Check sheet for the drawn part. Datum: minimum x, y, z corner. Units: mm. A direction names the side the tool comes from. Round coordinates to 2 decimals unless told otherwise and drop trailing zeros. Loops run counter-clockwise (first coordinate to the right, second up) from the corner with the lowest first, then second, coordinate; pieces in that order, holes last. Notation, with made-up numbers: (17.5, 22.25) -> (49.5, 22.25) arc R16 ccw to (49.5, 37.25) -> close; hole circle Ø7 at (-12.75, 1). An arc over 180 degrees is marked (long way). Return JSON: item names as keys, results as strings.
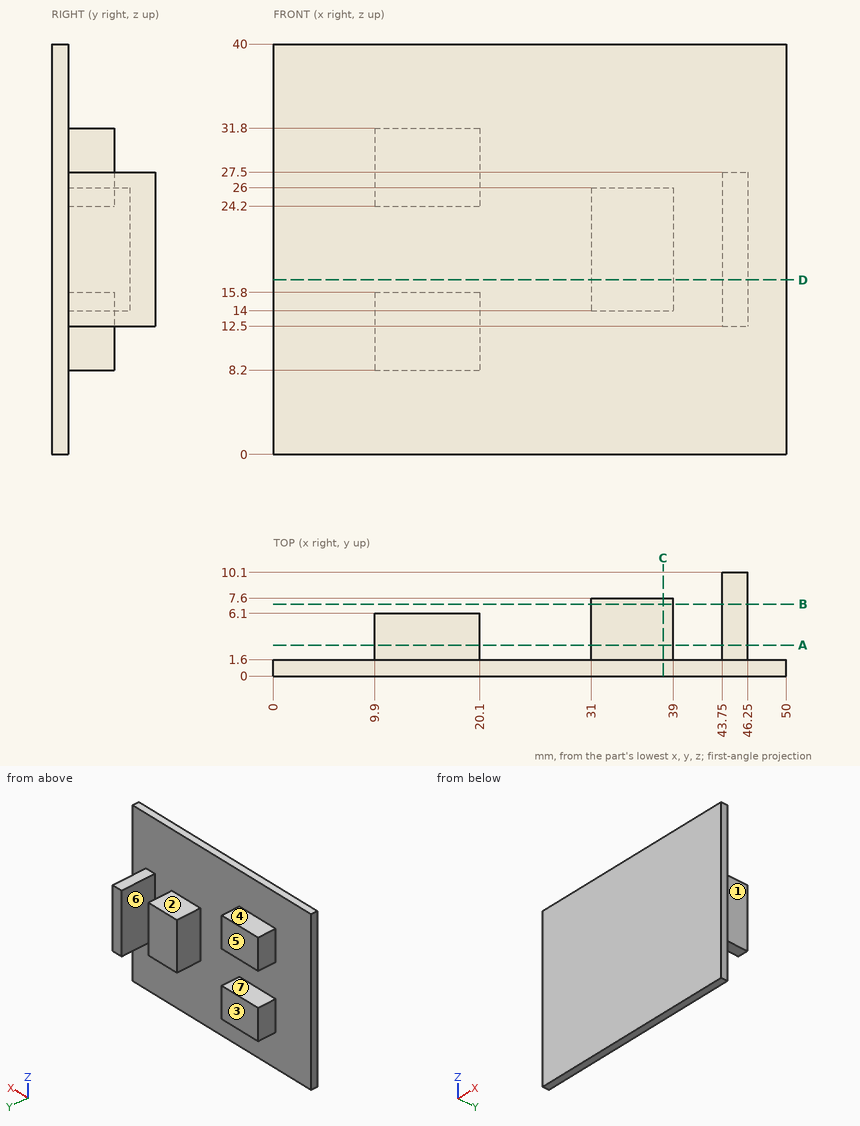
Q1. Go/stop test with flat-tipped pins: pin 1 (6 mm diameter, centred on x = 35.5, y = 7, fed in from +Z); pin 2 (6 mm diameter, centred on x = 15.5, z = 26.5, fed in from +Y); pin 3 (4 mm diameter, centred on y = 6, z = 22.5, fed in from -X). Record where each tip stops, or that it passes through.
Results list:
{"pin 1": "z = 26", "pin 2": "y = 6.1", "pin 3": "x = 9.9"}
Q2. Tool access check on the marked faces 4, 5, 6 and 7. Record the directions out of +Z, -Z, +X, -X, +Y, -Y that give a thin tool (end or side, any length) a straight path to the whole face; none if there is none.
Results list:
{"face 4": "+Z, +X, -X, +Y", "face 5": "+Z, -Z, -X, +Y", "face 6": "+Z, -Z, +Y", "face 7": "-X, +Y"}
Q3. Section check C-C (x = 38). Record the boundary of the cut face in (y, z).
Results list:
{"outline": "(0, 0) -> (1.6, 0) -> (1.6, 14) -> (7.6, 14) -> (7.6, 26) -> (1.6, 26) -> (1.6, 40) -> (0, 40) -> close"}
Q4. Draft check along X on the marked faces 1, 2 and 3. Enter one of: released by +X, released by -X, zero draft, split by the parting line, or undercut.
Results list:
{"face 1": "released by +X", "face 2": "undercut", "face 3": "zero draft"}
Q5. Section check A-A (y = 3). Record the boundary of the cut face in (x, z), then the cut area to 3 significant figures.
Results list:
{"outline": "(9.9, 8.2) -> (20.1, 8.2) -> (20.1, 15.8) -> (9.9, 15.8) -> close; (9.9, 24.2) -> (20.1, 24.2) -> (20.1, 31.8) -> (9.9, 31.8) -> close; (31, 14) -> (39, 14) -> (39, 26) -> (31, 26) -> close; (43.75, 12.5) -> (46.25, 12.5) -> (46.25, 27.5) -> (43.75, 27.5) -> close", "area": "289 mm^2"}
Q6. Material ranges on line 1 (X direction, y = 7.25, z = 19.5); line 2 (Y direction, x = 13, z = 8.5); line 3 (X direction, y = 5.5, z = 11.5), recorded low to high.
Results list:
{"line 1": "31 to 39, 43.75 to 46.25", "line 2": "0 to 6.1", "line 3": "9.9 to 20.1"}
Q7. Section check B-B (y = 7). Record the boundary of the cut face in (x, z), then the cut area to 4 significant figures.
Results list:
{"outline": "(31, 14) -> (39, 14) -> (39, 26) -> (31, 26) -> close; (43.75, 12.5) -> (46.25, 12.5) -> (46.25, 27.5) -> (43.75, 27.5) -> close", "area": "133.5 mm^2"}
Q8. Section check D-D (z = 17). Record the boundary of the cut face in (x, y).
Results list:
{"outline": "(0, 0) -> (50, 0) -> (50, 1.6) -> (46.25, 1.6) -> (46.25, 10.1) -> (43.75, 10.1) -> (43.75, 1.6) -> (39, 1.6) -> (39, 7.6) -> (31, 7.6) -> (31, 1.6) -> (0, 1.6) -> close"}
